from build123d import *

# Parameters (mm, degrees)
EXTRUDE_1_DEPTH     = 5
SKETCH_2_R          = 1.5
CUT_EXTRUDE_1_DEPTH = 5
SKETCH_3_R          = 1.5
CUT_EXTRUDE_2_DEPTH = 133.382022949


with BuildPart() as part:
    # 草图1 → 凸台-拉伸1 (new body)
    with BuildSketch(Plane.XY):
        Polygon((86.602540378, 50), (0, 100), (-86.602540378, 50), (-86.602540378, -50), (0, -100), (86.602540378, -50), align=None)
    extrude(amount=EXTRUDE_1_DEPTH)

    # 草图2 → 切除-拉伸1 (cut)
    with BuildSketch(Plane(origin=(0, 0, 0), x_dir=(-1, 0, 0), z_dir=(0, 0, -1))):
        with Locations((-81.602540378, 17.365)):
            Circle(SKETCH_2_R)
        with Locations((-62.002540378, 17.37)):
            Circle(SKETCH_2_R)
        with Locations(Location((-62.002540378, -17.37, 0), (0, 0, 180))):
            Circle(SKETCH_2_R)
        with Locations(Location((-81.602540378, -17.365, 0), (0, 0, 180))):
            Circle(SKETCH_2_R)
        with Locations((55.839801326, 61.987372981)):
            Circle(SKETCH_2_R)
        with Locations((46.044131453, 45.010775067)):
            Circle(SKETCH_2_R)
        with Locations(Location((15.958408925, 62.380775067, 0), (0, 0, 180))):
            Circle(SKETCH_2_R)
        with Locations(Location((25.762739053, 79.352372981, 0), (0, 0, 180))):
            Circle(SKETCH_2_R)
        with Locations((25.762739053, -79.352372981)):
            Circle(SKETCH_2_R)
        with Locations((15.958408925, -62.380775067)):
            Circle(SKETCH_2_R)
        with Locations(Location((46.044131453, -45.010775067, 0), (0, 0, 180))):
            Circle(SKETCH_2_R)
        with Locations(Location((55.839801326, -61.987372981, 0), (0, 0, 180))):
            Circle(SKETCH_2_R)
    extrude(amount=-CUT_EXTRUDE_1_DEPTH, mode=Mode.SUBTRACT)

    # 草图3 → 切除-拉伸2 (cut, through all)
    with BuildSketch(Plane.XY.offset(5)):
        Circle(SKETCH_3_R)
        with Locations((10, 0)):
            Circle(SKETCH_3_R)
        with Locations((20, 0)):
            Circle(SKETCH_3_R)
        with Locations((30, 0)):
            Circle(SKETCH_3_R)
        with Locations((40, 0)):
            Circle(SKETCH_3_R)
        with Locations((10, 10)):
            Circle(SKETCH_3_R)
        with Locations((20, 10)):
            Circle(SKETCH_3_R)
        with Locations((30, 10)):
            Circle(SKETCH_3_R)
        with Locations((40, 10)):
            Circle(SKETCH_3_R)
        with Locations((10, 20)):
            Circle(SKETCH_3_R)
        with Locations((20, 20)):
            Circle(SKETCH_3_R)
        with Locations((30, 20)):
            Circle(SKETCH_3_R)
        with Locations((40, 20)):
            Circle(SKETCH_3_R)
        with Locations((10, 30)):
            Circle(SKETCH_3_R)
        with Locations((20, 30)):
            Circle(SKETCH_3_R)
        with Locations((30, 30)):
            Circle(SKETCH_3_R)
        with Locations((40, 30)):
            Circle(SKETCH_3_R)
        with Locations((0, 10)):
            Circle(SKETCH_3_R)
        with Locations((0, 20)):
            Circle(SKETCH_3_R)
        with Locations((0, 30)):
            Circle(SKETCH_3_R)
        with Locations(Location((0, -30, 0), (0, 0, 180))):
            Circle(SKETCH_3_R)
        with Locations(Location((0, -20, 0), (0, 0, 180))):
            Circle(SKETCH_3_R)
        with Locations(Location((0, -10, 0), (0, 0, 180))):
            Circle(SKETCH_3_R)
        with Locations(Location((40, -30, 0), (0, 0, 180))):
            Circle(SKETCH_3_R)
        with Locations(Location((30, -30, 0), (0, 0, 180))):
            Circle(SKETCH_3_R)
        with Locations(Location((20, -30, 0), (0, 0, 180))):
            Circle(SKETCH_3_R)
        with Locations(Location((10, -30, 0), (0, 0, 180))):
            Circle(SKETCH_3_R)
        with Locations(Location((40, -20, 0), (0, 0, 180))):
            Circle(SKETCH_3_R)
        with Locations(Location((30, -20, 0), (0, 0, 180))):
            Circle(SKETCH_3_R)
        with Locations(Location((20, -20, 0), (0, 0, 180))):
            Circle(SKETCH_3_R)
        with Locations(Location((10, -20, 0), (0, 0, 180))):
            Circle(SKETCH_3_R)
        with Locations(Location((40, -10, 0), (0, 0, 180))):
            Circle(SKETCH_3_R)
        with Locations(Location((30, -10, 0), (0, 0, 180))):
            Circle(SKETCH_3_R)
        with Locations(Location((20, -10, 0), (0, 0, 180))):
            Circle(SKETCH_3_R)
        with Locations(Location((10, -10, 0), (0, 0, 180))):
            Circle(SKETCH_3_R)
        with Locations((-10, -10)):
            Circle(SKETCH_3_R)
        with Locations((-20, -10)):
            Circle(SKETCH_3_R)
        with Locations((-30, -10)):
            Circle(SKETCH_3_R)
        with Locations((-40, -10)):
            Circle(SKETCH_3_R)
        with Locations((-10, -20)):
            Circle(SKETCH_3_R)
        with Locations((-20, -20)):
            Circle(SKETCH_3_R)
        with Locations((-30, -20)):
            Circle(SKETCH_3_R)
        with Locations((-40, -20)):
            Circle(SKETCH_3_R)
        with Locations((-10, -30)):
            Circle(SKETCH_3_R)
        with Locations((-20, -30)):
            Circle(SKETCH_3_R)
        with Locations((-30, -30)):
            Circle(SKETCH_3_R)
        with Locations((-40, -30)):
            Circle(SKETCH_3_R)
        with Locations(Location((-40, 30, 0), (0, 0, 180))):
            Circle(SKETCH_3_R)
        with Locations(Location((-30, 30, 0), (0, 0, 180))):
            Circle(SKETCH_3_R)
        with Locations(Location((-20, 30, 0), (0, 0, 180))):
            Circle(SKETCH_3_R)
        with Locations(Location((-10, 30, 0), (0, 0, 180))):
            Circle(SKETCH_3_R)
        with Locations(Location((-40, 20, 0), (0, 0, 180))):
            Circle(SKETCH_3_R)
        with Locations(Location((-30, 20, 0), (0, 0, 180))):
            Circle(SKETCH_3_R)
        with Locations(Location((-20, 20, 0), (0, 0, 180))):
            Circle(SKETCH_3_R)
        with Locations(Location((-10, 20, 0), (0, 0, 180))):
            Circle(SKETCH_3_R)
        with Locations(Location((-40, 10, 0), (0, 0, 180))):
            Circle(SKETCH_3_R)
        with Locations(Location((-30, 10, 0), (0, 0, 180))):
            Circle(SKETCH_3_R)
        with Locations(Location((-20, 10, 0), (0, 0, 180))):
            Circle(SKETCH_3_R)
        with Locations(Location((-10, 10, 0), (0, 0, 180))):
            Circle(SKETCH_3_R)
        with Locations(Location((-40, 0, 0), (0, 0, 180))):
            Circle(SKETCH_3_R)
        with Locations(Location((-30, 0, 0), (0, 0, 180))):
            Circle(SKETCH_3_R)
        with Locations(Location((-20, 0, 0), (0, 0, 180))):
            Circle(SKETCH_3_R)
        with Locations(Location((-10, 0, 0), (0, 0, 180))):
            Circle(SKETCH_3_R)
    extrude(amount=-CUT_EXTRUDE_2_DEPTH, mode=Mode.SUBTRACT)


solid = part.part
Work out the finished part from the listing and answer in its coordinate system (mm). Round coordinates to 2 decimals unless told otherwise and drop trailing zeros. Loops run counter-clockwise (first coordinate to the right, second up) from the corner with the lowest first, then second, coordinate; pieces in that order, holes last. Notation, with made-up numbers: M 64,16.25 L 90,16.25 A24 ccw 90,33.25 Z; hole C 16.5,44.25 d1. An arc over 180 degrees is marked long. One line per question, with ' | ' between items. Start each with the question number.
(1) Flat-ended cylindrical pins translate along their axes: pin 1 Ø4 at (x, y) = (10, 30) entering from +Z; pin 2 Ø2.5 at (x, y) = (20, -20) entering from +Z; pin 3 Ø1.5 at (y, z) = (-74, 2.5) entering from -X. Find the tip coordinate at first contact, or state that the pin passes through.
(2) A cutting plane is placed at B-B on x = 53. Write down the section's boundary in (y, z), plus the area to 3 significant figures.
(3) A cutting plane is placed at A-A on z = 0.95. Give the number of separate pieces and of enclosed holes in the cut face, plus the area to 3 significant figures.
(4) Find the intervals of material crossed by line 1 (X direction, y = 45.5, z = 0.2); line 2 (Y direction, x = 78, z = 4.45); line 3 (X direction, y = 87, z = 2.2), in increasing order.
(5) A cutting plane is placed at C-C on y = -85. Write down the section's boundary in (x, z), plus the area to 3 significant figures.
Geometry check:
1) pin 1: stops at z = 5 | pin 2: passes through | pin 3: stops at x = -46.33
2) outline: M -69.4,0 L 69.4,0 L 69.4,5 L -69.4,5 Z | area: 694 mm²
3) separate pieces: 1 | enclosed holes: 75 | area: 25,500 mm²
4) line 1: x = -86.6 to -47.46, -44.63 to 86.6 | line 2: y = -54.97 to 54.97 | line 3: x = -22.52 to 22.52
5) outline: M -25.98,0 L 25.98,0 L 25.98,5 L -25.98,5 Z | area: 260 mm²
